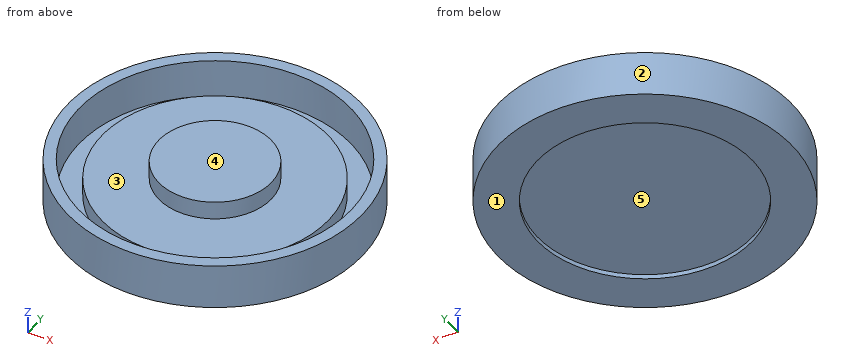
Autodesk Inventor part; units mm, degrees
ref_plane "YZ Plane" through (0, 0, 0) normal (1, 0, 0) x (0, 1, 0)
ref_plane "XZ Plane" through (0, 0, 0) normal (0, 1, 0) x (-1, 0, 0)
ref_plane "XY Plane" through (0, 0, 0) normal (0, 0, 1) x (1, 0, 0)
sketch "Skizze1" plane through (0, 0, 0) normal (0, 0, 1) x (1, 0, 0)
  circle A0 centre (0, 0) radius 6.5
  dimension "d2" = 13
extrude "Extrusion1" add sketch "Skizze1" along normal blind 2
sketch "Skizze2" plane through (0, 0, 2) normal (0, 0, 1) x (1, 0, 0)
  circle A0 centre (0, 0) radius 6
  dimension "d3" = 12
extrude "Extrusion2" cut sketch "Skizze2" against normal blind 1.7
sketch "Skizze3" plane through (0, 0, 0.3) normal (0, 0, 1) x (1, 0, 0)
  circle A0 centre (0, 0) radius 5
  dimension "d6" = 10
extrude "Extrusion3" add sketch "Skizze3" along normal blind 0.8
sketch "Skizze4" plane through (0, 0, 1.1) normal (0, 0, 1) x (1, 0, 0)
  circle A0 centre (0, 0) radius 2.4903
extrude "Extrusion4" add sketch "Skizze4" along normal blind 0.8
sketch "Skizze5" plane through (0, 0, 0) normal (0, 0, -1) x (-1, 0, 0)
  circle A0 centre (0, 0) radius 4.75
  dimension "d11" = 9.5
extrude "Extrusion5" cut sketch "Skizze5" against normal blind 0.2
properties part number "Gummipad" material "Glas"
CAD build for the part. Positions are in the model's coordinates, mm. Face numbers are marked on the shaded views. A direction names the side the tool comes from. Give positions to 0.01 mm unless a question says otherwise; leave off trailing zeros. Write each loop counter-clockwise with the first axis right and the second up, starting at its lowest first coordinate (ties: lowest second). Pieces come first, ordered by that corner, then holes. Notation, with made-up numbers: (-10.75, 88) -> (30.25, 88) arc R30 ccw to (30.25, 125) -> close; hole circle Ø3 at (80, 88.5). An arc over 180 degrees is marked (long way). Return JSON: item names as keys, results as strings.
Item 1: Drill centre lines: probe 1 along Y at (x, z) = (0, 0.75); probe 2 along Y at (x, z) = (0, 0.15); probe 3 along Y at (x, z) = (0, 1.55). Where is each one in solid material? Low to high.
Answer below:
{"probe 1": "y = -6.5 to -6, -5 to 5, 6 to 6.5", "probe 2": "y = -6.5 to -4.75, 4.75 to 6.5", "probe 3": "y = -6.5 to -6, -2.49 to 2.49, 6 to 6.5"}
Item 2: Two-plate mould, pull along Y, no slides. Class the marked faces 1, 2 and 3: +Y half, -Y half, draft (parallel to the pull), parting line (faces both ways), or undercut.
Answer below:
{"face 1": "draft", "face 2": "parting line", "face 3": "undercut"}
Item 3: Tool access for the marked faces 4 and 5: list every direction of +Z, -Z, +X, -X, +Y, -Y with a clear straight run to the whole face (end or side of a thin tool).
Answer below:
{"face 4": "+Z", "face 5": "-Z"}
Item 4: Band-saw the part on A-A (y = 0). List the corners of the cut face in (x, z), then the cut area to 3 significant figures.
Answer below:
{"outline": "(-6.5, 0) -> (-4.75, 0) -> (-4.75, 0.2) -> (4.75, 0.2) -> (4.75, 0) -> (6.5, 0) -> (6.5, 2) -> (6, 2) -> (6, 0.3) -> (5, 0.3) -> (5, 1.1) -> (2.49, 1.1) -> (2.49, 1.9) -> (-2.49, 1.9) -> (-2.49, 1.1) -> (-5, 1.1) -> (-5, 0.3) -> (-6, 0.3) -> (-6, 2) -> (-6.5, 2) -> close", "area": "15.7 mm2"}
Item 5: Drop flat-ended pins along their axis: pin 1 (5.5 mm diameter, centred on x = 1, y = -0.5, fed in from +Z); pin 2 (1 mm diameter, centred on x = -0.5, z = 0.5, fed in from +Y); pin 3 (1 mm diameter, centred on x = 3.5, z = 1, fed in from +Y). Give the stop position or say it passes through.
Answer below:
{"pin 1": "stops at z = 1.9", "pin 2": "stops at y = 6.5", "pin 3": "stops at y = 5.77"}
Item 6: Band-saw the part on D-D (y = 4.5). List the corners of the cut face in (x, z), then the cut area to 3 significant figures.
Answer below:
{"outline": "(-4.69, 0) -> (-1.52, 0) -> (-1.52, 0.2) -> (1.52, 0.2) -> (1.52, 0) -> (4.69, 0) -> (4.69, 2) -> (3.97, 2) -> (3.97, 0.3) -> (2.18, 0.3) -> (2.18, 1.1) -> (-2.18, 1.1) -> (-2.18, 0.3) -> (-3.97, 0.3) -> (-3.97, 2) -> (-4.69, 2) -> close", "area": "8.15 mm2"}
Item 7: Band-saw the part on B-B (z = 0.95). List the corners of the cut face in (x, y), then the cut area to 3 significant figures.
Answer below:
{"outline": "circle Ø13 at (0, 0); circle Ø10 at (0, 0); hole circle Ø12 at (0, 0)", "area": "98.2 mm2"}
